from build123d import *

# Parameters (mm, degrees)
SKETCH1_W           = 115
SKETCH1_H           = 33
BOSS_EXTRUDE1_DEPTH = 24
SKETCH2_W           = 5
SKETCH2_H           = 24
BOSS_EXTRUDE2_DEPTH = 15
SKETCH3_W           = 17
SKETCH3_H           = 24
SKETCH3_W_2         = 15
BOSS_EXTRUDE3_DEPTH = 7


with BuildPart() as part:
    # Sketch1 → Boss-Extrude1 (new body)
    with BuildSketch(Plane(origin=(0, 0, 0), x_dir=(1, 0, 0), z_dir=(0, 1, 0))):
        Rectangle(SKETCH1_W, SKETCH1_H)
    extrude(amount=BOSS_EXTRUDE1_DEPTH)

    # Sketch2 → Boss-Extrude2 (add)
    with BuildSketch(Plane.ZY.offset(57.5)):
        with Locations((14, 12)):
            Rectangle(SKETCH2_W, SKETCH2_H)
    extrude(amount=BOSS_EXTRUDE2_DEPTH)

    # Sketch3 → Boss-Extrude3 (add)
    with BuildSketch(Plane.XY.offset(16.5)):
        with Locations((-49, 12)):
            Rectangle(SKETCH3_W, SKETCH3_H)
        with Locations((-65, 12)):
            Rectangle(SKETCH3_W_2, SKETCH3_H)
    extrude(amount=BOSS_EXTRUDE3_DEPTH)


solid = part.part
The listing builds one solid part. Answer for the finished solid, in the listing's coordinates (mm). A direction names the side the tool comes from. Coordinates: 2 decimals unless noted, no trailing zeros. Loops run counter-clockwise (first coordinate to the right, second up) from the corner with the lowest first, then second, coordinate; pieces in that order, holes last. Notation, with made-up numbers: (68, 45.5) -> (73, 45.5) arc R20 ccw to (73, 51.5) -> close; hole circle Ø9 at (20.25, 3.5). An arc over 180 degrees is marked (long way). Answer in a Markdown table with one row per item. Add a question column.
1. The part is cut by section A-A, the plane y = 22. Write down the section's boundary in (x, z).
2. For faces 1 (the flat face through (-40.5, 12, 20)), 2 (the flat face through (-8, 0, -1)), 3 (the flat face through (-57.5, 12, -2)), determine the directions among +Z, -Z, +X, -X, +Y, -Y from which every point of the face is accessible in a straight line to the end or side of a thin tool.
3. Flat-ended cylindrical pins translate along their axes: P1, Ø5, axis at y = 14, z = -4, coming from the -X side; P2, Ø4.5, axis at x = -66, y = 10.5, coming from the -Z side; P3, Ø3.5, axis at y = 9, z = 18.5, coming from the +X side. Find the tip coordinate at first contact, or state that the pin passes through.
4. Consider line 1 (X direction, y = 2, z = 2); line 2 (Z direction, x = -18, y = 7.5); line 3 (Z direction, x = -64.5, y = 5.5). Determine where each line is inside the solid, lowest interval first. Write a range as [from, to].
5. The part is cut by section C-C, the plane x = 12.5. Write down the section's boundary in (y, z).
6. The part is cut by section B-B, the plane z = -9. Write down the section's boundary in (x, y), then the cut area to 3 significant figures.
Answer below:
| question | item | result |
|---|---|---|
| 1 | outline | (-72.5, 11.5) -> (-57.5, 11.5) -> (-57.5, -16.5) -> (57.5, -16.5) -> (57.5, 16.5) -> (-40.5, 16.5) -> (-40.5, 23.5) -> (-72.5, 23.5) -> close |
| 2 | face 1 | +Z, +X, +Y, -Y |
| 2 | face 2 | +Z, -Z, +X, -X, -Y |
| 2 | face 3 | -Z, -X, +Y, -Y |
| 3 | P1 | x = -57.5 |
| 3 | P2 | z = 11.5 |
| 3 | P3 | x = -40.5 |
| 4 | line 1 | [-57.5, 57.5] |
| 4 | line 2 | [-16.5, 16.5] |
| 4 | line 3 | [11.5, 23.5] |
| 5 | outline | (0, -16.5) -> (24, -16.5) -> (24, 16.5) -> (0, 16.5) -> close |
| 6 | outline | (-57.5, 0) -> (57.5, 0) -> (57.5, 24) -> (-57.5, 24) -> close |
| 6 | area | 2,760 mm2 |
